Model file for the job. Use its own axes, mm. Give positions to 0.01 mm unless a question says otherwise; leave off trailing zeros. Return JSON: item names as keys, results as strings. Group by question number.
1. Slice it at A-A on z = 4. Give the number of separate pieces and of enclosed holes in the cut face, then the cut area to 3 significant figures.
2. Wall check: probe 1 along X at (y, z) = (-34, 4.5); probe 2 along X at (y, z) = (-28.5, 9.5); probe 3 along X at (y, z) = (-46.5, 12.25). Give the ranges that are in metal, low to high. Write a range as [from, to].
3. Pin check, flat tip, straight feed: pin 1 (10.5 mm diameter, centred on x = 195.57, y = -6.38, fed in from -Z). Stop position of the tip, or through.
Autodesk Inventor part; units mm, degrees
ref_plane "YZ Plane" through (0, 0, 0) normal (1, 0, 0) x (0, 1, 0)
ref_plane "XZ Plane" through (0, 0, 0) normal (0, 1, 0) x (-1, 0, 0)
ref_plane "XY Plane" through (0, 0, 0) normal (0, 0, 1) x (1, 0, 0)
sketch "Sketch1" plane through (0, 0, 0) normal (0, 0, 1) x (1, 0, 0)
  line L0 (246.3741, 31.7234) -> (246.3741, -882.6766) construction
  line L1 (234.1821, 31.7234) -> (231.3881, 31.7234) construction
  line L2 (223.2601, 31.7234) -> (220.4661, 31.7234) construction
  line L3 (199.5111, 31.7234) -> (196.0821, 31.7234) construction
  line L4 (182.3661, 31.7234) -> (178.9371, 31.7234) construction
  line L5 (246.3741, 31.7234) -> (170.1741, 31.7234)
  line L6 (170.1741, 31.7234) -> (170.1741, -69.8766)
  line L7 (170.1741, -69.8766) -> (246.3741, -69.8766)
  line L8 (246.3741, -69.8766) -> (246.3741, 31.7234)
  circle A0 centre (227.3241, 15.8484) radius 3.9688
  line L9 (208.2741, -69.8766) -> (208.2741, 31.7234) construction
  line L10 (246.3741, -19.0766) -> (170.1741, -19.0766) construction
  circle A1 centre (227.3241, -54.0016) radius 3.9688
  circle A2 centre (189.2241, 15.8484) radius 3.9688
  circle A3 centre (189.2241, -54.0016) radius 3.9688
  point P0 (0, 0)
  dimension "d0" = 76.2
  dimension "d1" = 101.6
  dimension "d2" = 7.9375
  dimension "d3" = 15.875
  dimension "d4" = 19.05
extrude "Extrusion1" add sketch "Sketch1" along normal blind 12.7
sketch "Sketch3" plane through (0, 0, 0) normal (0, 0, -1) x (-1, 0, 0)
  line L0 (-186.0491, -41.3016) -> (-230.4991, -41.3016)
  line L1 (-230.4991, -41.3016) -> (-230.4991, 3.1484)
  line L2 (-230.4991, 3.1484) -> (-186.0491, 3.1484)
  line L3 (-186.0491, 3.1484) -> (-186.0491, -41.3016)
  line L4 (-170.1741, -69.8766) -> (-246.3741, -69.8766)
  line L5 (-170.1741, 31.7234) -> (-170.1741, -69.8766)
  line L6 (-246.3741, 31.7234) -> (-170.1741, 31.7234)
  circle A0 centre (-195.5741, -6.3766) radius 6.35
  circle A1 centre (-195.5741, -31.7766) radius 6.35
  circle A2 centre (-220.9741, -6.3766) radius 6.35
  circle A3 centre (-220.9741, -31.7766) radius 6.35
  point P0 (0, 0)
  dimension "d16" = 44.45
  dimension "d17" = 44.45
  dimension "d18" = 28.575
  dimension "d19" = 15.875
  dimension "d23" = 12.7
  dimension "d24" = 9.525
  dimension "d25" = 9.525
  dimension "d28" = 25.4
  dimension "d31" = 25.4
extrude "Extrusion3" cut sketch "Sketch3" against normal blind 7.9375 contours A0 | A1 | A2 | A3
sketch "Sketch4" plane through (195.5741, -6.3766, 7.9375) normal (0, 0, -1) x (-1, 0, 0)
  circle A0 centre (0, 0) radius 6.35
  circle A1 centre (0, -25.4) radius 6.35
  circle A2 centre (-25.4, 0) radius 6.35
  circle A3 centre (-25.4, -25.4) radius 6.35
  circle A4 centre (0, 0) radius 3.9688
  line L0 (0, 0) -> (0, -11.1628) construction
  line L1 (0, 0) -> (-15.7699, 0) construction
  circle A5 centre (0, -25.4) radius 3.9688
  circle A6 centre (-25.4, 0) radius 3.9688
  circle A7 centre (-25.4, -25.4) radius 3.9688
  point P0 (195.5741, 6.3766)
  dimension "d36" = 7.9375
  dimension "d37" = 7.9375
  dimension "d38" = 7.9375
  dimension "d39" = 7.9375
extrude "Extrusion4" cut sketch "Sketch4" against normal blind 7.9375 contours A4 | A5 | A6 | A7
sketch "Sketch5" plane through (0, 0, 12.7) normal (0, 0, 1) x (1, 0, 0)
  line L0 (589.2741, -69.8766) -> (589.2741, 844.5234)
  line L1 (246.3741, -69.8766) -> (589.2741, -69.8766)
  line L2 (246.3741, 31.7234) -> (170.1741, 31.7234)
  line L3 (246.3741, 31.7234) -> (589.2741, 31.7234)
  line L4 (376.7143, 0.5706) -> (376.7143, -56.5544)
  line L5 (376.7143, 18.2956) -> (376.7143, 9.7706)
  line L6 (376.7143, 18.2956) -> (376.7143, 23.7956)
  line L7 (376.7143, -62.0544) -> (376.7143, -56.5544)
  circle A0 centre (227.3241, 15.8484) radius 3.9688
  circle A1 centre (227.3241, -54.0016) radius 3.9688
  circle A2 centre (570.2241, 18.2956) radius 3.9688
  circle A3 centre (570.2241, -50.0328) radius 3.9688
  line L8 (246.3741, 31.7234) -> (246.3741, -69.8766)
  point P0 (0, 0)
  dimension "d42" = 7.9375
  dimension "d43" = 7.9375
  dimension "d44" = 19.05
  dimension "d45" = 19.05
extrude "Extrusion5" add sketch "Sketch5" against normal blind 12.7 contours L1 L8 L3 L0
properties part number "Corner Stands"
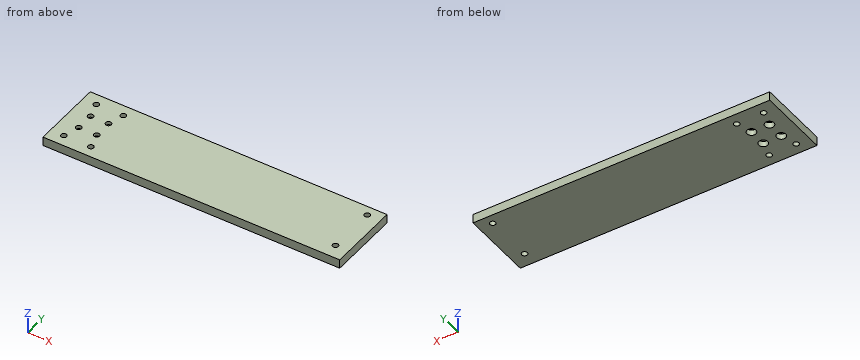
Result:
{
 "1": {"separate pieces": "1", "enclosed holes": "10", "area": "41,800 mm2"},
 "2": {"probe 1": "x = [170.17, 189.63], [201.52, 215.03], [226.92, 589.27]", "probe 2": "x = [170.17, 193.33], [197.81, 218.73], [223.21, 589.27]", "probe 3": "x = [170.17, 568.42], [572.03, 589.27]"},
 "3": {"pin 1": "stops at z = 7.94"}
}
